Autodesk Inventor part; units mm, degrees
ref_plane "YZ Plane" through (0, 0, 0) normal (1, 0, 0) x (0, 1, 0)
ref_plane "XZ Plane" through (0, 0, 0) normal (0, 1, 0) x (-1, 0, 0)
ref_plane "XY Plane" through (0, 0, 0) normal (0, 0, 1) x (1, 0, 0)
sketch "Sketch1" plane through (0, 0, 0) normal (0, 1, 0) x (-1, 0, 0)
  line L0 (6.35, -3.6662) -> (0, -7.3323)
  line L1 (0, -7.3323) -> (-6.35, -3.6662)
  line L2 (-6.35, -3.6662) -> (-6.35, 3.6662)
  line L3 (-6.35, 3.6662) -> (0, 7.3323)
  line L4 (0, 7.3323) -> (6.35, 3.6662)
  line L5 (6.35, 3.6662) -> (6.35, -3.6662)
  point P0 (0, 0)
  point P1 (0, 0)
  point P2 (0, 0)
  dimension "d0" = 12.7
extrude "Extrusion1" add sketch "Sketch1" along normal blind 532.4348
sketch "Sketch2" plane through (0, 0, 0) normal (0, -1, 0) x (1, 0, 0)
  point P0 (0, 0)
  point P1 (0, 0)
hole "Hole1" at (0, 0, 0) direction (0, 1, 0) diameter 4.9784 depth 25.4
sketch "Sketch3" plane through (0, 532.4348, 0) normal (0, 1, 0) x (1, 0, 0)
  point P0 (0, 0)
  point P1 (0.0338, 0.0857)
hole "Hole2" at (0.0338, 532.4348, -0.0857) direction (0, -1, 0) diameter 4.9784 depth 25.4
properties part number "INTK_003_HexShaft5" material "Aluminum 7075"
Verification items for the finished model (mm, model axes). Coordinates: 2 decimals unless noted, no trailing zeros. Write each loop counter-clockwise with the first axis right and the second up, starting at its lowest first coordinate (ties: lowest second). Pieces come first, ordered by that corner, then holes. Notation, with made-up numbers: M 4,23 L 20,23 A30 cw 20,47 Z; hole C 56,77 d4. An arc over 180 degrees is marked long. Answer as a JSON object with one key per item and string values. Group by question number.
(1) Cross-section at A-A, the plane y = 95.5. Record the cut outline in (x, z), and give its area (3 significant figures).
(2) Material ranges on line 1 (X direction, y = 11, z = 0); line 2 (Z direction, x = 0, y = 17); line 3 (Y direction, x = -1.5, z = 0.75), recorded low to high.
(3) Gauge pin test, flat ends, axial feed: pin 1 (2 mm diameter, centred on x = 0.5, y = 431, fed in from -Z); pin 2 (6 mm diameter, centred on x = 4, y = 76, fed in from -Z); pin 3 (1.5 mm diameter, centred on x = -2, y = 456.5, fed in from +Z). Record the tip position at first contact, or that the pin passes through.
(4) Cross-section at B-B, the plane z = 0. Record the cut outline in (x, y), and give its area (3 significant figures).
Reply:
{
 "1": {"outline": "M -6.35,-3.67 L 0,-7.33 L 6.35,-3.67 L 6.35,3.67 L 0,7.33 L -6.35,3.67 Z", "area": "140 mm²"},
 "2": {"line 1": "-6.35 to -2.49, 2.49 to 6.35", "line 2": "-7.33 to -2.49, 2.49 to 7.33", "line 3": "25.4 to 507.03"},
 "3": {"pin 1": "z = -7.33", "pin 2": "z = -6.75", "pin 3": "z = 6.61"},
 "4": {"outline": "M -6.35,0 L -2.49,0 L -2.49,25.4 L 2.49,25.4 L 2.49,0 L 6.35,0 L 6.35,532.43 L 2.52,532.43 L 2.52,507.03 L -2.45,507.03 L -2.45,532.43 L -6.35,532.43 Z", "area": "6,510 mm²"}
}
